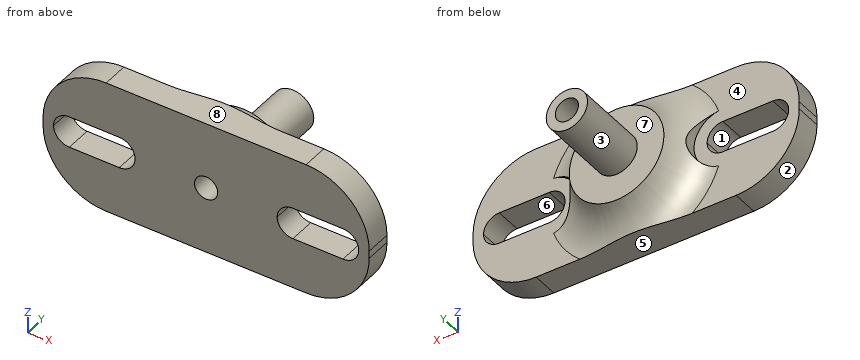
```python
from build123d import *

# Parameters (mm, degrees)
SKETCH1_W           = 62
SKETCH1_H           = 25.4
SKETCH1_R           = 3.925
SKETCH1_W_2         = 15.5
SKETCH1_H_2         = 6
BOSS_EXTRUDE1_DEPTH = 5
SKETCH1_3_R         = 3.925
SKETCH1_3_R_2       = 2.2
BOSS_EXTRUDE2_DEPTH = 24.5
FILLET1_R           = 3
SKETCH2_R           = 9
BOSS_EXTRUDE3_DEPTH = 5.5
FILLET2_R           = 8
SKETCH3_R           = 5.5
CUT_EXTRUDE1_DEPTH  = 5.5
FILLET3_R           = 12
SKETCH4_R           = 2.2
CUT_EXTRUDE2_DEPTH  = 42.503493918


# Some blends are built 0.0001 mm under size
with BuildPart() as part:
    # Sketch1 → Boss-Extrude1 (new body)
    with BuildSketch(Plane(origin=(0, 0, 0), x_dir=(1, 0, 0), z_dir=(0, 1, 0))):
        Rectangle(SKETCH1_W, SKETCH1_H)
        with Locations(Location((0, 0, 0), (0, 0, 270))):
            Circle(SKETCH1_R, mode=Mode.SUBTRACT)
        with Locations((-21.25, 0)):
            Rectangle(SKETCH1_W_2, SKETCH1_H_2, mode=Mode.SUBTRACT)
        with Locations((21.25, 0)):
            Rectangle(SKETCH1_W_2, SKETCH1_H_2, mode=Mode.SUBTRACT)
    extrude(amount=BOSS_EXTRUDE1_DEPTH)

    # Sketch1<3> → Boss-Extrude2 (add)
    with BuildSketch(Plane(origin=(0, 0, 0), x_dir=(1, 0, 0), z_dir=(0, 1, 0))):
        with Locations(Location((0, 0, 0), (0, 0, 270))):
            Circle(SKETCH1_3_R)
        with Locations(Location((0, 0, 0), (0, 0, 270))):
            Circle(SKETCH1_3_R_2, mode=Mode.SUBTRACT)
    extrude(amount=BOSS_EXTRUDE2_DEPTH)

    # Fillet1
    fillet1_edges = [part.edges().sort_by_distance(p)[0] for p in [
        (29, 2.5, 3),
        (13.5, 2.5, 3),
        (29, 2.5, -3),
        (13.5, 2.5, -3),
        (-29, 2.5, 3),
        (-29, 2.5, -3),
        (-13.5, 2.5, 3),
        (-13.5, 2.5, -3),
    ]]
    fillet(fillet1_edges, radius=FILLET1_R - 0.0001)  # a hair under: the kernel refuses the full size

    # Sketch2 → Boss-Extrude3 (add)
    with BuildSketch(Plane(origin=(0, 5, 0), x_dir=(1, 0, 0), z_dir=(0, 1, 0))):
        with Locations(Location((0, 0, 0), (0, 0, 270))):
            Circle(SKETCH2_R)
    extrude(amount=BOSS_EXTRUDE3_DEPTH)

    # Fillet2
    # the kernel refuses this fillet: 8 mm, written as the material it adds along each edge
    with BuildSketch(Plane(origin=(0, 5, 0), x_dir=(0, 0, 1), z_dir=(-1, 0, 0))) as fillet2_piece_1_section:
        with BuildLine():
            CenterArc((16.599342077, 8), FILLET2_R, 198.209956864, 71.790043136)
            Line((9, 5.5), (9, 0))
            Line((9, 0), (16.599342077, 0))
        make_face()
    fillet2_piece_1 = revolve(axis=Axis((0, 5, 0), (0, 1, 0)), mode=Mode.PRIVATE)
    fillet2_piece_1 = fillet2_piece_1 - Plane(origin=(-16.4999, 5, -0.0001), x_dir=(0, 0, -1), z_dir=(0, 1, 0)) * Cylinder(2.9999, 67, mode=Mode.PRIVATE)
    fillet2_piece_1 = split(fillet2_piece_1, bisect_by=Plane(origin=(0, 5, 12.7), z_dir=(0, 0, -1)), keep=Keep.TOP, mode=Mode.PRIVATE)
    fillet2_piece_1 = split(fillet2_piece_1, bisect_by=Plane(origin=(0, 5, -12.7), z_dir=(0, 0, 1)), keep=Keep.TOP, mode=Mode.PRIVATE)
    fillet2_piece_1 = fillet2_piece_1 - Plane(origin=(16.4999, 5, 0.0001), x_dir=(0, 0, 1), z_dir=(0, 1, 0)) * Cylinder(2.9999, 67, mode=Mode.PRIVATE)
    add(fillet2_piece_1)

    # Sketch3 → Cut-Extrude1 (cut)
    with BuildSketch(Plane(origin=(0, 5, 0), x_dir=(1, 0, 0), z_dir=(0, 1, 0))):
        with Locations((16.5, 0)):
            Circle(SKETCH3_R)
        with Locations((-16.5, 0)):
            Circle(SKETCH3_R)
    extrude(amount=CUT_EXTRUDE1_DEPTH, mode=Mode.SUBTRACT)

    # Fillet3
    fillet3_edges = [part.edges().sort_by_distance(p)[0] for p in [
        (-31, 2.5, 12.7),
        (-31, 2.5, -12.7),
        (31, 2.5, -12.7),
        (31, 2.5, 12.7),
    ]]
    fillet(fillet3_edges, radius=FILLET3_R)

    # Sketch4 → Cut-Extrude2 (cut, through all)
    with BuildSketch(Plane(origin=(0, 24.5, 0), x_dir=(1, 0, 0), z_dir=(0, 1, 0))):
        with Locations(Location((0, 0, 0), (0, 0, 270))):
            Circle(SKETCH4_R)
    extrude(amount=-CUT_EXTRUDE2_DEPTH, mode=Mode.SUBTRACT)


solid = part.part
```
For this review, take the finished solid that the model builds, in its own axes (mm). Face numbers are marked on the shaded views. A direction names the side the tool comes from. Coordinates: 2 decimals unless noted, no trailing zeros. Write each loop counter-clockwise with the first axis right and the second up, starting at its lowest first coordinate (ties: lowest second). Pieces come first, ordered by that corner, then holes. Notation, with made-up numbers: (16.5, -23.75) -> (24.5, -23.75) arc R24 ccw to (24.5, -13.75) -> close; hole circle Ø11 at (48.25, 80.25). An arc over 180 degrees is marked (long way). Put each result on its own line as item: value.
Q1. Take a section at D-D, the plane y = 16.5. State the section outline as (x, z) points (3 decimals).
From the geometry:
outline: circle Ø7.85 at (0, 0); hole circle Ø4.4 at (0, 0)
Q2. Clearance check with flat-ended pins moving along their axes: pin 1 Ø10 at (x, y) = (0.5, 17) entering from -Z (3 decimals); pin 2 Ø8 at (x, y) = (15.5, 13) entering from -Z; pin 3 Ø8 at (x, z) = (-7, 8) entering from +Y; pin 4 Ø10 at (x, z) = (21.5, -5) entering from +Y. State where each tip first meets the part, or that it passes through.
From the geometry:
pin 1: stops at z = -3.925
pin 2: passes through
pin 3: stops at y = 10.5
pin 4: stops at y = 5
Q3. Tool access review of the marked faces 1, 2, 3, 4 and 5: name each direction out of +Z, -Z, +X, -X, +Y, -Y from which nothing blocks a thin tool from reaching the whole face with its end or side.
From the geometry:
face 1: +Y, -Y
face 2: -Z, -X, +Y, -Y
face 3: +Y
face 4: -X, +Y
face 5: -Z, +X, -X, +Y, -Y
Q4. Wall thickness on L1, parallel to X at y = 12.75, z = 0 (3 decimals); L2, parallel to Y at x = -14, z = 2.5; L3, parallel to Y at x = -3, z = -2.75: over which ranges is each line inside the solid? List them lowest first.
From the geometry:
L1: x = -3.925 to -2.2, 2.2 to 3.925
L2: y = 0 to 5
L3: y = 0 to 10.5
Q5. Take a section at A-A, the plane x = 0. State the section outline as (y, z) points (3 decimals), then the cut area to 3 significant figures.
From the geometry:
outline: (0, -12.7) -> (6.015, -12.7) arc R8 cw to (10.5, -9) -> (10.5, -3.925) -> (24.5, -3.925) -> (24.5, -2.2) -> (0, -2.2) -> close; (0, 2.2) -> (24.5, 2.2) -> (24.5, 3.925) -> (10.5, 3.925) -> (10.5, 9) arc R8 cw to (6.015, 12.7) -> (0, 12.7) -> close
area: 248 mm2
Q6. Take a section at B-B, the plane y = 3.5. Count the separate pieces of the cut face and the enclosed holes in it, then the cut area to 3 significant figures.
From the geometry:
separate pieces: 1
enclosed holes: 3
area: 1,270 mm2
Q7. Take a section at C-C, the plane x = 18. State the section outline as (y, z) points, then the cut area to 3 significant figures.
From the geometry:
outline: (0, -12.7) -> (5, -12.7) -> (5, -3) -> (0, -3) -> close; (0, 3) -> (5, 3) -> (5, 12.7) -> (0, 12.7) -> close
area: 97.0 mm2
Q8. The part is to be moulded in two halves that separate along Z. For the marked faces 6, 7 and 8, say which applies: +Z half, -Z half, draft (parallel to the pull), parting line (faces both ways), or undercut.
From the geometry:
face 6: undercut
face 7: draft
face 8: +Z half
